Design review of the part built by this model. Coordinates are the model's own, in mm. Face numbers are marked on the shaded views. A direction names the side the tool comes from. Round coordinates to 2 decimals unless told otherwise and drop trailing zeros. Write each loop counter-clockwise with the first axis right and the second up, starting at its lowest first coordinate (ties: lowest second). Pieces come first, ordered by that corner, then holes. Notation, with made-up numbers: (34.5, -20.75) - (50.5, -20.75) arc R29 cw to (50.5, 12.25) - close; hole circle Ø11 at (-29.75, -2.5). An arc over 180 degrees is marked (long way). Use one line per item in the form item = value.
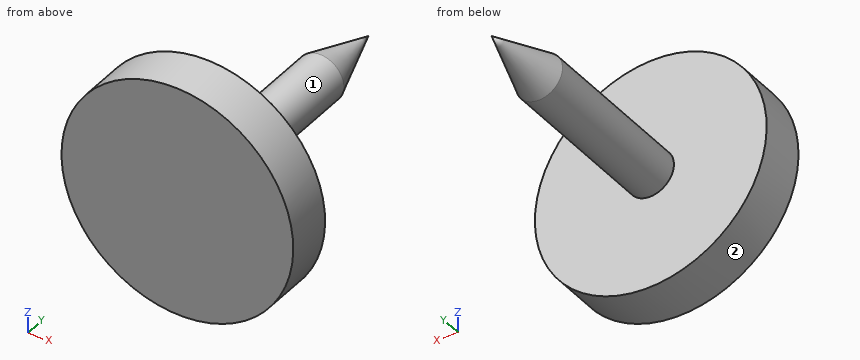
```python
from build123d import *

# Parameters (mm, degrees)
SKETCH_2_R      = 50
EXTRUDE_1_DEPTH = 20
SKETCH_3_R      = 10
EXTRUDE_2_DEPTH = 70


with BuildPart() as part:
    # 草图2 → 凸台-拉伸1 (new body)
    with BuildSketch(Plane(origin=(0, 0, 0), x_dir=(1, 0, 0), z_dir=(0, 1, 0))):
        with Locations(Location((0, 0, 0), (0, 0, 270))):
            Circle(SKETCH_2_R)
    extrude(amount=EXTRUDE_1_DEPTH)

    # 草图3 → 凸台-拉伸2 (add)
    with BuildSketch(Plane(origin=(0, 20, 0), x_dir=(1, 0, 0), z_dir=(0, 1, 0))):
        with Locations(Location((0, 0, 0), (0, 0, 270))):
            Circle(SKETCH_3_R)
    extrude(amount=EXTRUDE_2_DEPTH)

    # 草图4 → 旋转1 (revolve)
    with BuildSketch(Plane.XY, mode=Mode.PRIVATE) as revolve_1_sk:
        Polygon((0, 90), (10, 90), (0, 120), align=None)
    revolve(revolve_1_sk.sketch.rotate(Axis((0, 0, 0), (0, 1, 0)), 90), axis=Axis((0, 0, 0), (0, 1, 0)))


solid = part.part
```
Q1. We need section B-B on x = 34. Write out the cut boundary in (y, z).
Calculated:
outline = (0, -36.66) - (20, -36.66) - (20, 36.66) - (0, 36.66) - close
Q2. To check wall thickness, follow line 1 along Y through (x, z) = (-26.5, 15); line 2 along X through (y, z) = (6, -18); line 3 along X through (y, z) = (12, -27). State the ranges of each line that lie inside material, in increasing order. Write a range as from..to.
Calculated:
line_1 = 0..20
line_2 = -46.65..46.65
line_3 = -42.08..42.08
Q3. We need section C-C on z = 37.5. Write out the cut boundary in (x, y).
Calculated:
outline = (-33.07, 0) - (33.07, 0) - (33.07, 20) - (-33.07, 20) - close
Q4. Machinability: for the marked faces 1 and 2, which of the approach directions +Z, -Z, +X, -X, +Y, -Y give a long, thin tool a straight path to every point of the face, cutting with its end or side? Answer none if there is none.
Calculated:
face_1 = +Y
face_2 = +Y, -Y
Q5. For P1, Ø6, axis at x = -6.5, y = 41, coming from the +Z side; P2, Ø8, axis at y = 93.5, z = -5.5, coming from the -X side, all flat-tipped, find the tip position at first contact; note any pin that passes through.
Calculated:
P1 = 9.37
P2 = -9.41
Q6. We need section A-A on y = 32.5. Write out the cut boundary in (x, z), then the cut area to 3 significant figures.
Calculated:
outline = circle Ø20 at (0, 0)
area = 314 mm2
